```python
from build123d import *

# Parameters (mm, degrees)
SKETCH1_R                     = 22.5
SKETCH1_R_2                   = 12.5
SKETCH1_R_3                   = 1.7
SKETCH1_R_4                   = 20
SKETCH1_R_5                   = 11.5
BOSS_EXTRUDE1_DEPTH           = 5
SKETCH2_R                     = 3
CUT_EXTRUDE1_DEPTH            = 2
SKETCH3_R                     = 13
SKETCH3_R_2                   = 11.5
BOSS_EXTRUDE2_DEPTH           = 3.5
SKETCH4_R                     = 11.5
SKETCH4_R_2                   = 10
BOSS_EXTRUDE3_DEPTH           = 1
BOSS_EXTRUDE4_DEPTH           = 3.5
CHAMFER1_SIZE                 = 2.5
CHAMFER1_SIZE2                = 4.160698706
CIRPATTERN1_COUNT             = 6
CHAMFER1_OF_CIRPATTERN1_SIZE2 = 2.5
CHAMFER1_OF_CIRPATTERN1_SIZE  = 4.160698706
SKETCH7_W                     = 16
SKETCH7_H                     = 5
BOSS_EXTRUDE5_DEPTH           = 5


with BuildPart() as part:
    # Sketch1 → Boss-Extrude1 (new body)
    # profile 1 of 9: a face of its own
    with BuildSketch(Plane(origin=(0, 0, 0), x_dir=(1, 0, 0), z_dir=(0, 1, 0))):
        Circle(SKETCH1_R)
        with Locations(Location((0, 0, 0), (0, 0, 270))):
            Circle(SKETCH1_R_2, mode=Mode.SUBTRACT)
        with Locations(Location((-15.588457268, 9, 0), (0, 0, 270))):
            Circle(SKETCH1_R_3, mode=Mode.SUBTRACT)
        with Locations(Location((-15.588457268, -9, 0), (0, 0, 270))):
            Circle(SKETCH1_R_3, mode=Mode.SUBTRACT)
        with Locations(Location((0, -18, 0), (0, 0, 270))):
            Circle(SKETCH1_R_3, mode=Mode.SUBTRACT)
        with Locations(Location((15.588457268, -9, 0), (0, 0, 270))):
            Circle(SKETCH1_R_3, mode=Mode.SUBTRACT)
        with Locations(Location((15.588457268, 9, 0), (0, 0, 270))):
            Circle(SKETCH1_R_3, mode=Mode.SUBTRACT)
        with Locations(Location((0, 18, 0), (0, 0, 270))):
            Circle(SKETCH1_R_3, mode=Mode.SUBTRACT)
    # profile 2 of 9: a face of its own
    with BuildSketch(Plane(origin=(0, 0, 0), x_dir=(1, 0, 0), z_dir=(0, 1, 0))):
        with BuildLine():
            Line((100.5, 19.993749023), (0.5625, 22.492967651))
            ThreePointArc((0.5625, 22.492967651), (9.388247907, 20.447757854), (16.691908913, 15.087417832))
            Line((16.691908913, 15.087417832), (18.813128873, 15.034370753))
            Line((18.813128873, 15.034370753), (79.921396282, 13.506186436))
            Line((79.921396282, 13.506186436), (85.131066178, 13.375903969))
            ThreePointArc((85.131066178, 13.375903969), (92.090162259, 18.3693894), (100.5, 19.993749023))
        make_face()
    # profile 3 of 9: a face of its own
    with BuildSketch(Plane(origin=(0, 0, 0), x_dir=(1, 0, 0), z_dir=(0, 1, 0))):
        with BuildLine():
            Line((18.813128873, 15.034370753), (16.691908913, 15.087417832))
            ThreePointArc((16.691908913, 15.087417832), (18.903398529, 12.202930961), (20.621590627, 9))
            Line((20.621590627, 9), (44.334992825, 0))
            Line((44.334992825, 0), (51.380509764, 2.674000631))
            Line((51.380509764, 2.674000631), (18.813128873, 15.034370753))
        make_face()
    # profile 4 of 9: a face of its own
    with BuildSketch(Plane(origin=(0, 0, 0), x_dir=(1, 0, 0), z_dir=(0, 1, 0))):
        Polygon((58.426026703, 0), (51.380509764, 2.674000631), (44.334992825, 0), (51.380509764, -2.674000631), align=None)
    # profile 5 of 9: a face of its own
    with BuildSketch(Plane(origin=(0, 0, 0), x_dir=(1, 0, 0), z_dir=(0, 1, 0))):
        with BuildLine():
            ThreePointArc((82.139428901, 9), (83.489631833, 11.287503843), (85.131066178, 13.375903969))
            Line((85.131066178, 13.375903969), (79.921396282, 13.506186436))
            Line((79.921396282, 13.506186436), (51.380509764, 2.674000631))
            Line((51.380509764, 2.674000631), (58.426026703, 0))
            Line((58.426026703, 0), (82.139428901, 9))
        make_face()
    # profile 6 of 9: a face of its own
    with BuildSketch(Plane(origin=(0, 0, 0), x_dir=(1, 0, 0), z_dir=(0, 1, 0))):
        with BuildLine():
            Line((79.921396282, -13.506186436), (85.131066178, -13.375903969))
            ThreePointArc((85.131066178, -13.375903969), (83.489631833, -11.287503843), (82.139428901, -9))
            Line((82.139428901, -9), (58.426026703, 0))
            Line((58.426026703, 0), (51.380509764, -2.674000631))
            Line((51.380509764, -2.674000631), (79.921396282, -13.506186436))
        make_face()
    # profile 7 of 9: a face of its own
    with BuildSketch(Plane(origin=(0, 0, 0), x_dir=(1, 0, 0), z_dir=(0, 1, 0))):
        with BuildLine():
            ThreePointArc((20.621590627, -9), (18.903398529, -12.202930961), (16.691908913, -15.087417832))
            Line((16.691908913, -15.087417832), (18.813128873, -15.034370753))
            Line((18.813128873, -15.034370753), (51.380509764, -2.674000631))
            Line((51.380509764, -2.674000631), (44.334992825, 0))
            Line((44.334992825, 0), (20.621590627, -9))
        make_face()
    # profile 8 of 9: a face of its own
    with BuildSketch(Plane(origin=(0, 0, 0), x_dir=(1, 0, 0), z_dir=(0, 1, 0))):
        with BuildLine():
            ThreePointArc((16.691908913, -15.087417832), (9.388247907, -20.447757854), (0.5625, -22.492967651))
            Line((0.5625, -22.492967651), (100.5, -19.993749023))
            ThreePointArc((100.5, -19.993749023), (92.090162259, -18.3693894), (85.131066178, -13.375903969))
            Line((85.131066178, -13.375903969), (79.921396282, -13.506186436))
            Line((79.921396282, -13.506186436), (18.813128873, -15.034370753))
            Line((18.813128873, -15.034370753), (16.691908913, -15.087417832))
        make_face()
    # profile 9 of 9: a face of its own
    with BuildSketch(Plane(origin=(0, 0, 0), x_dir=(1, 0, 0), z_dir=(0, 1, 0))):
        with Locations((100, 0)):
            Circle(SKETCH1_R_4)
        with Locations(Location((86.143593539, 8, 0), (0, 0, 270))):
            Circle(SKETCH1_R_3, mode=Mode.SUBTRACT)
        with Locations(Location((86.143593539, -8, 0), (0, 0, 270))):
            Circle(SKETCH1_R_3, mode=Mode.SUBTRACT)
        with Locations(Location((100, -16, 0), (0, 0, 270))):
            Circle(SKETCH1_R_3, mode=Mode.SUBTRACT)
        with Locations(Location((113.856406461, -8, 0), (0, 0, 270))):
            Circle(SKETCH1_R_3, mode=Mode.SUBTRACT)
        with Locations(Location((113.856406461, 8, 0), (0, 0, 270))):
            Circle(SKETCH1_R_3, mode=Mode.SUBTRACT)
        with Locations(Location((100, 16, 0), (0, 0, 270))):
            Circle(SKETCH1_R_3, mode=Mode.SUBTRACT)
        with Locations(Location((100, 0, 0), (0, 0, 270))):
            Circle(SKETCH1_R_5, mode=Mode.SUBTRACT)
    extrude(amount=BOSS_EXTRUDE1_DEPTH)

    # Sketch2 → Cut-Extrude1 (cut)
    with BuildSketch(Plane(origin=(0, 5, 0), x_dir=(1, 0, 0), z_dir=(0, 1, 0))):
        with Locations(Location((0, 18, 0), (0, 0, 270))):
            Circle(SKETCH2_R)
        with Locations(Location((-15.588457268, -9, 0), (0, 0, 270))):
            Circle(SKETCH2_R)
        with Locations(Location((15.588457268, -9, 0), (0, 0, 270))):
            Circle(SKETCH2_R)
        with Locations(Location((100, 16, 0), (0, 0, 270))):
            Circle(SKETCH2_R)
        with Locations(Location((86.143593539, -8, 0), (0, 0, 270))):
            Circle(SKETCH2_R)
        with Locations(Location((113.856406461, -8, 0), (0, 0, 270))):
            Circle(SKETCH2_R)
    extrude(amount=-CUT_EXTRUDE1_DEPTH, mode=Mode.SUBTRACT)

    # Sketch3 → Boss-Extrude2 (add)
    with BuildSketch(Plane(origin=(0, 5, 0), x_dir=(1, 0, 0), z_dir=(0, 1, 0))):
        with Locations(Location((100, 0, 0), (0, 0, 90))):
            Circle(SKETCH3_R)
        with Locations(Location((100, 0, 0), (0, 0, 270))):
            Circle(SKETCH3_R_2, mode=Mode.SUBTRACT)
    extrude(amount=BOSS_EXTRUDE2_DEPTH)

    # Sketch4 → Boss-Extrude3 (add)
    with BuildSketch(Plane.XZ):
        with Locations(Location((100, 0, 0), (0, 0, 270))):
            Circle(SKETCH4_R)
        with Locations(Location((100, 0, 0), (0, 0, 270))):
            Circle(SKETCH4_R_2, mode=Mode.SUBTRACT)
    extrude(amount=-BOSS_EXTRUDE3_DEPTH)

    # Sketch6 → Boss-Extrude4 (add)
    with BuildSketch(Plane(origin=(0, 5, 0), x_dir=(1, 0, 0), z_dir=(0, 1, 0))):
        with BuildLine():
            Line((87.08682843, 1.5), (82.5, 1.5))
            Line((82.5, 1.5), (82.5, -1.5))
            Line((82.5, -1.5), (87.08682843, -1.5))
            ThreePointArc((87.08682843, -1.5), (87, 0), (87.08682843, 1.5))
        make_face()
    boss_extrude4 = extrude(amount=BOSS_EXTRUDE4_DEPTH)

    # Chamfer1
    chamfer1_edges = [part.edges().sort_by_distance(p)[0] for p in [
        (82.5, 8.5, 0),
    ]]
    chamfer1_side = [part.faces().sort_by_distance(p)[0] for p in [
        (82.5, 6.75, 0),
    ]]
    chamfer(chamfer1_edges, length=CHAMFER1_SIZE, length2=CHAMFER1_SIZE2, reference=chamfer1_side[0])

    # CirPattern1: Boss-Extrude4 ×6 about axis
    cirpattern1_axis = Axis((100, 0, 0), (0, 1, 0))
    for i in range(1, CIRPATTERN1_COUNT):
        add(boss_extrude4.rotate(cirpattern1_axis, i * 360 / CIRPATTERN1_COUNT))

    # Chamfer1 of CirPattern1
    chamfer1_of_cirpattern1_edges = [part.edges().sort_by_distance(p)[0] for p in [
        (91.25, 8.5, 15.155444566),
        (108.75, 8.5, 15.155444566),
        (117.5, 8.5, 0),
        (108.75, 8.5, -15.155444566),
        (91.25, 8.5, -15.155444566),
    ]]
    chamfer(chamfer1_of_cirpattern1_edges, length=CHAMFER1_OF_CIRPATTERN1_SIZE, length2=CHAMFER1_OF_CIRPATTERN1_SIZE2)

    # Sketch7 → Boss-Extrude5 (add)
    with BuildSketch(Plane.XZ):
        with Locations((-30, 0)):
            Rectangle(SKETCH7_W, SKETCH7_H)
    extrude(amount=-BOSS_EXTRUDE5_DEPTH)


solid = part.part
```
Input: part model. Units: mm. Frame: model coordinates. A direction names the side the tool comes from. Round coordinates to 2 decimals unless told otherwise and drop trailing zeros. Answer in a Markdown table with one row per item. Add a question column.
1. Ray query, probe 1 along Z at (x, y) = (34, 2.5); probe 2 along X at (y, z) = (4.55, -18); probe 3 along Z at (x, y) = (74, 2). Return the intervals inside material, ascending.
2. Set-up query: faces 5 (the face through (65.451, 2.465, 8.014)), 6 (the face through (-2, 3, -18)), 7 (the face through (111.295, 6.726, -6.436)), 8 (the face through (-30, 2, -2.5)), 9 (the face through (-30, 2, 2.5)). Return all of +Z, -Z, +X, -X, +Y, -Y with unobstructed straight access to the full face (end or side cutting, diameter ignored); none if empty.
3. Contact query for flat-ended pins moving along their axis: pin 1 (1.5 mm diameter, centred on y = 7, z = 9, fed in from -X); pin 2 (3 mm diameter, centred on x = 87, z = 9.5, fed in from +Y); pin 3 (1 mm diameter, centred on x = 84.5, y = 7.5, fed in from -Z). Output: stop coordinate, or through.
4. Mould query, pull axis Z, two halves, no side actions, for faces 1 (the face through (90, 8.5, 6)), 2 (the face through (-0.65, 1.48, -16.43)), 3 (the face through (120, 2, 0)), 4 (the face through (85, 6, -1.5)). Classes: released by +Z, released by -Z, zero draft, split by the parting line, or undercut.
Values follow:
| question | item | result |
|---|---|---|
| 1 | probe 1 | -21.66 to -14.65, -9.27 to -3.92, 3.92 to 9.27, 14.65 to 21.66 |
| 1 | probe 2 | -13.5 to -3, 3 to 97.76, 102.24 to 108.72 |
| 1 | probe 3 | -20.66 to -13.65, -11.26 to -5.91, 5.91 to 11.26, 13.65 to 20.66 |
| 2 | face 5 | +Y, -Y |
| 2 | face 6 | +Y |
| 2 | face 7 | +X, +Y |
| 2 | face 8 | -Z, -X, +Y, -Y |
| 2 | face 9 | +Z, -X, +Y, -Y |
| 3 | pin 1 | x = 89.95 |
| 3 | pin 2 | y = 5 |
| 3 | pin 3 | z = -1.5 |
| 4 | face 1 | zero draft |
| 4 | face 2 | undercut |
| 4 | face 3 | split by the parting line |
| 4 | face 4 | released by -Z |
